Can you work these out from the model? Positions are in its coordinate system, mm. Face numbers are marked on the shaded views. Coordinates: 2 decimals unless noted, no trailing zeros. Order: outer loops, then holes, each group sorted by start corner. A loop starts at its lowest first (then second) coordinate and runs counter-clockwise, first axis right, second up.
```python
from build123d import *

# Parameters (mm, degrees)
SKETCH1_W                = 23.025
SKETCH1_H                = 15
SKETCH2_R                = 22.575
BOSS_EXTRUDE1_DEPTH      = 13
HOLE1_D                  = 20
HOLE1_CBORE_D            = 28
HOLE1_CBORE_DEPTH        = 27
M2_CLEARANCE_HOLE1_D     = 2.459
M2_CLEARANCE_HOLE1_DEPTH = 14.999999999
M2_CLEARANCE_HOLE1_TIP   = 0.738758131


with BuildPart() as part:
    # Sketch1 → Revolve1 (revolve)
    with BuildSketch(Plane(origin=(0, 0, 0), x_dir=(1, 0, 0), z_dir=(0, 1, 0))):
        with Locations((11.5125, -20.5)):
            Rectangle(SKETCH1_W, SKETCH1_H)
    revolve(axis=Axis((0, 0, 13), (0, 0, 1)))

    # Sketch2 → Boss-Extrude1 (add)
    with BuildSketch(Plane(origin=(0, 0, 13), x_dir=(-1, 0, 0), z_dir=(0, 0, -1))):
        with Locations(Location((0, 0, 0), (0, 0, 180))):
            Circle(SKETCH2_R)
    extrude(amount=BOSS_EXTRUDE1_DEPTH)

    # Hole1 (through all)
    with Locations(Plane.XY.offset(28)):
        with Locations((0, 0)):
            CounterBoreHole(HOLE1_D / 2, HOLE1_CBORE_D / 2, HOLE1_CBORE_DEPTH)

    # M2 Clearance Hole1
    with Locations(Plane(origin=(0, 0, 0), x_dir=(-1, 0, 0), z_dir=(0, 0, -1))):
        with Locations((0, 17.5), (-17.5, 0), (0, -17.5), (17.5, 0)):
            Hole(M2_CLEARANCE_HOLE1_D / 2, depth=M2_CLEARANCE_HOLE1_DEPTH)
            with Locations((0, 0, -(M2_CLEARANCE_HOLE1_DEPTH + M2_CLEARANCE_HOLE1_TIP / 2))):  # 118° drill point
                Cone(0, M2_CLEARANCE_HOLE1_D / 2, M2_CLEARANCE_HOLE1_TIP, mode=Mode.SUBTRACT)


solid = part.part
```
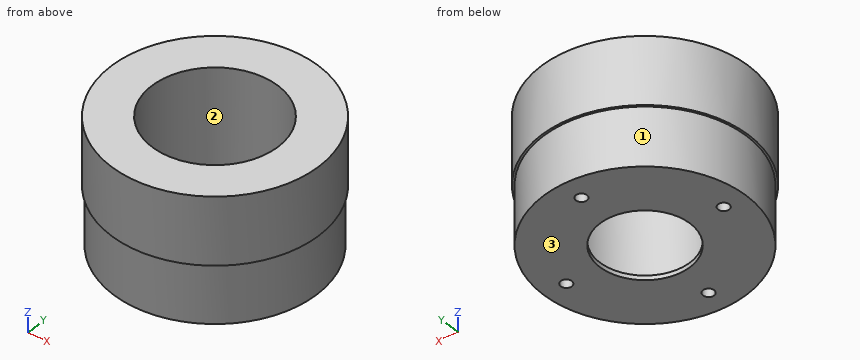
1. I'm going to push flat-ended pins straight in: pin 1 (1 mm diameter, centred on y = 16.5, z = 24, fed in from -X); pin 2 (2 mm diameter, centred on x = -17.5, y = 0, fed in from -Z); pin 3 (10 mm diameter, centred on x = 0.5, z = 21, fed in from -Y) (3 decimals); pin 4 (14 mm diameter, centred on x = -2, y = 0, fed in from +Z). Where does each tip first touch, or does it pass through?
Completed:
pin 1: stops at x = -16.56
pin 2: stops at z = 15.14
pin 3: stops at y = -23.025
pin 4: passes through
2. Imagine slicing it at B-B on x = -9. Please give me the cut outline in (y, z).
Completed:
outline: (-21.19, 13) - (-20.7, 13) - (-20.7, 0) - (-4.36, 0) - (-4.36, 1) - (-10.72, 1) - (-10.72, 28) - (-21.19, 28) - close; (4.36, 0) - (20.7, 0) - (20.7, 13) - (21.19, 13) - (21.19, 28) - (10.72, 28) - (10.72, 1) - (4.36, 1) - close
3. Imagine slicing it at A-A on y = -7.5. Please give me the cut outline in (x, z).
Completed:
outline: (-21.77, 13) - (-21.29, 13) - (-21.29, 0) - (-6.61, 0) - (-6.61, 1) - (-11.82, 1) - (-11.82, 28) - (-21.77, 28) - close; (6.61, 0) - (21.29, 0) - (21.29, 13) - (21.77, 13) - (21.77, 28) - (11.82, 28) - (11.82, 1) - (6.61, 1) - close
4. Please list where these lines run through material, in increasing order: probe 1 along Y at (x, z) = (0.5, 4.75); probe 2 along X at (y, z) = (-1.5, 9.25); probe 3 along Y at (x, z) = (-7, 20.75).
Completed:
probe 1: y = -22.57 to -18.62, -16.38 to -13.99, 13.99 to 16.38, 18.62 to 22.57
probe 2: x = -22.53 to -13.92, 13.92 to 22.53
probe 3: y = -21.94 to -12.12, 12.12 to 21.94
5. Imagine slicing it at C-C on z = 5.75. Give the number of separate pieces and of enclosed holes in the cut face, then the cut area to 3 significant figures.
Completed:
separate pieces: 1
enclosed holes: 5
area: 966 mm2
6. Thinking about a two-plate mould opening in X: for the marked faces 1, 2 and 3, which applies, pulls with the +X half, pulls with the -X half, needs draft (parallel to the pull), parting line crosses it, or undercut?
Completed:
face 1: parting line crosses it
face 2: undercut
face 3: needs draft
7. Imagine slicing it at D-D on x = 12. Please give me the cut outline in (y, z).
Completed:
outline: (-19.65, 13) - (-19.12, 13) - (-19.12, 0) - (19.12, 0) - (19.12, 13) - (19.65, 13) - (19.65, 28) - (7.21, 28) - (7.21, 1) - (-7.21, 1) - (-7.21, 28) - (-19.65, 28) - close
